Design review of the part built by this model. Coordinates are the model's own, in mm. Give positions to 0.01 mm unless a question says otherwise; leave off trailing zeros. Loops run counter-clockwise (first coordinate to the right, second up) from the corner with the lowest first, then second, coordinate; pieces in that order, holes last. Notation, with made-up numbers: (-24, 40) - (29, 40) arc R20 cw to (29, 46) - close; hole circle Ø2 at (54.5, 4). An arc over 180 degrees is marked (long way). Put each result on its own line as item: value. Start each with the question number.
```python
from build123d import *

# Parameters (mm, degrees)
F1_DEPTH = 12


with BuildPart() as f1:
    # F0 (on Top) → F1 (new body)
    with BuildSketch(Plane.XY):
        with BuildLine():
            ThreePointArc((-19.687827, 18.926671), (-23.780217, 17.808299), (-27.363122, 20.080126))
            Line((-27.363122, 20.080126), (-31.07146, 13.657096))
            ThreePointArc((-31.07146, 13.657096), (-27.585511, 12.006069), (-26.168584, 8.418584))
            ThreePointArc((-26.168584, 8.418584), (-26.185187, 8.001384), (-26.234891, 7.586823))
            Line((-26.234891, 7.586823), (-25.080382, 6.920266))
            Line((-25.080382, 6.920266), (-18.533317, 18.260114))
            Line((-18.533317, 18.260114), (-19.687827, 18.926671))
        make_face()
    extrude(amount=F1_DEPTH)


solid = f1.part
```
Item 1: Consider section B-B (x = -30). State the section outline as (y, z) points.
Item 2: Mouldability with a two-part tool opening along X and no side actions: class faces 1 (the flat face through (-19.102, 18.589, 5.916)), 2 (the flat face through (-29.2, 16.9, 5.9)), 3 (the cylindrical face through (-23.72, 17.8, 5.92)), 4 (the flat face through (-25, 15, 0)) as pulls with the +X half, pulls with the -X half, needs draft (parallel to the pull), parting line crosses it, or undercut.
Item 3: Consider section C-C (y = 15.75). State the section outline as (x, z) points, plus the area to 3 significant figures.
Item 4: Consider section A-A (z = 10.5). State the section outline as (x, y) points.
Item 5: For L1, parallel to Y at x = -27.25, z = 9.5; L2, parallel to X at y = 13, z = 3; L3, parallel to Y at x = -20, z = 6.5, list the stretches that pass through material, from the lowest coordinate up. Write a range as from..to.
Item 6: For P1, Ø4, axis at y = 10, z = 4.5, coming from the +X side, flat-tipped, find the tip position at first contact; note if it passes through.
Geometry says:
1. outline: (13.47, 0) - (15.51, 0) - (15.51, 12) - (13.47, 12) - close
2. face 1: pulls with the +X half
2. face 2: pulls with the -X half
2. face 3: undercut
2. face 4: needs draft
3. outline: (-29.86, 0) - (-19.98, 0) - (-19.98, 12) - (-29.86, 12) - close
3. area: 119 mm2
4. outline: (-31.07, 13.66) arc R5.25 cw to (-26.17, 8.42) arc R5.25 cw to (-26.23, 7.59) - (-25.08, 6.92) - (-18.53, 18.26) - (-19.69, 18.93) arc R5.25 cw to (-27.36, 20.08) - close
5. L1: y = 11.61..19.92
5. L2: x = -28.85..-21.57
5. L3: y = 15.72..18.69
6. P1: stops at x = -22.15
